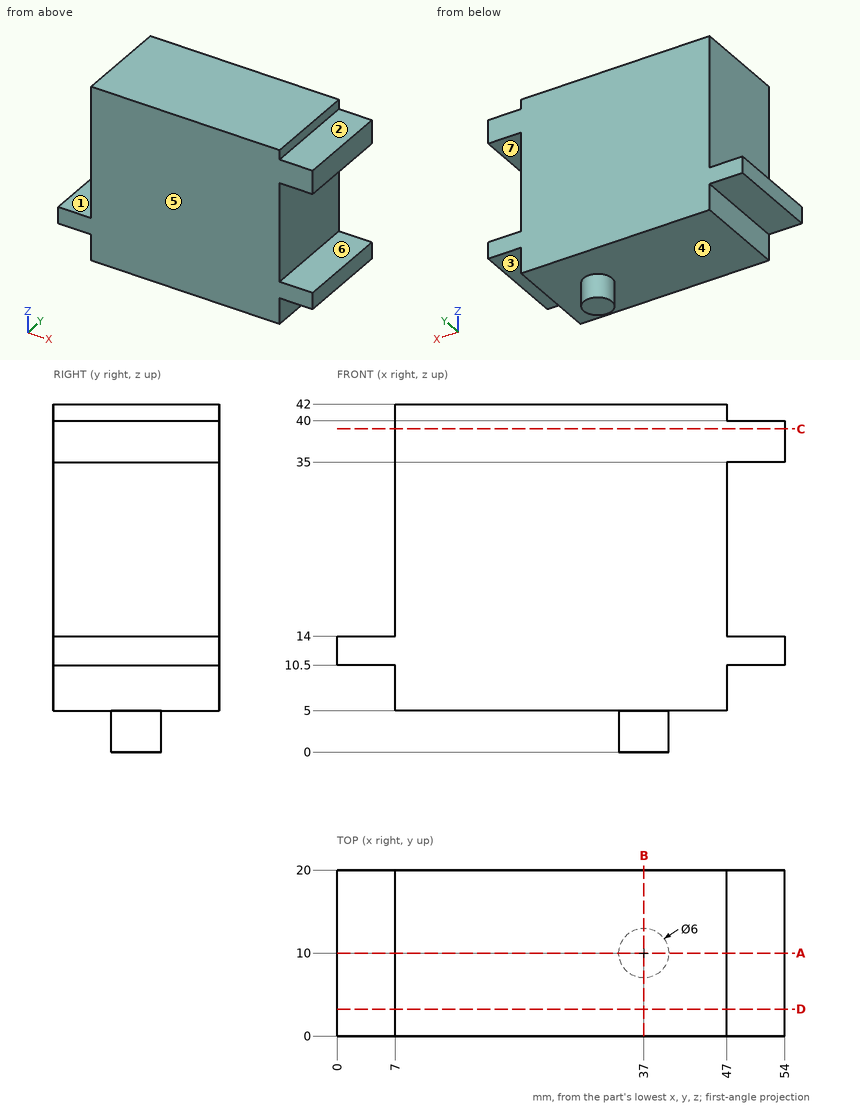
Answer from the drawing. Dimensions are ordinates in mm from the lowest x, y and z of the part. A direction names the side the tool comes from. Coordinates: 2 decimals unless noted, no trailing zeros. Write each loop counter-clockwise with the first axis right and the second up, starting at its lowest first coordinate (ties: lowest second). Pieces come first, ordered by that corner, then holes. Notation, with made-up numbers: M -25.75,-34 L -18.75,-34 A32 cw -18.75,0 Z; hole C 82.5,-20.5 d1. An arc over 180 degrees is marked long. Use a Markdown table: item, result.
Q1. The part is cut by section A-A, the plane y = 10. Write down the section's boundary in (x, z).
Answer block:
| item | result |
|---|---|
| outline | M 0,10.5 L 7,10.5 L 7,5 L 34,5 L 34,0 L 40,0 L 40,5 L 47,5 L 47,10.5 L 54,10.5 L 54,14 L 47,14 L 47,35 L 54,35 L 54,40 L 47,40 L 47,42 L 7,42 L 7,14 L 0,14 Z |
Q2. Determine the mould class of the marked faces 4, 5, 6 and 7 for opening direction Z: released by +Z, released by -Z, zero draft, split by the parting line, or undercut.
Answer block:
| item | result |
|---|---|
| face 4 | released by -Z |
| face 5 | zero draft |
| face 6 | undercut |
| face 7 | undercut |
Q3. The part is cut by section D-D, the plane y = 3.25. Write down the section's boundary in (x, z), then the cut area to 3 significant figures.
Answer block:
| item | result |
|---|---|
| outline | M 0,10.5 L 7,10.5 L 7,5 L 47,5 L 47,10.5 L 54,10.5 L 54,14 L 47,14 L 47,35 L 54,35 L 54,40 L 47,40 L 47,42 L 7,42 L 7,14 L 0,14 Z |
| area | 1,560 mm2 |
Q4. Each of these flat-tipped pins is pushed along its axis until it touches: pin 1 Ø3.5 at (x, y) = (51.5, 11) entering from +Z; pin 2 Ø1 at (x, y) = (38.5, 3) entering from -Z; pin 3 Ø1.6 at (y, z) = (13.5, 8.5) entering from +X. Where does it stop, or does it pass through?
Answer block:
| item | result |
|---|---|
| pin 1 | stops at z = 40 |
| pin 2 | stops at z = 5 |
| pin 3 | stops at x = 47 |
Q5. Which of the six approach directions +Z, -Z, +X, -X, +Y, -Y give full straight-line access (tool end or side, diameter ignored) to the marked faces 1, 2 and 3?
Answer block:
| item | result |
|---|---|
| face 1 | +Z, -X, +Y, -Y |
| face 2 | +Z, +X, +Y, -Y |
| face 3 | -Z, +X, +Y, -Y |
Q6. Straight lines are drawn through the part: L1, parallel to Z at x = 48.5, y = 10.5; L2, parallel to X at y = 14.25, z = 33; L3, parallel to Z at x = 27.5, y = 13. For each, find the intervals that lie inside material, in ascending order. Write a range as [from, to].
Answer block:
| item | result |
|---|---|
| L1 | z = [10.5, 14], [35, 40] |
| L2 | x = [7, 47] |
| L3 | z = [5, 42] |
Q7. The part is cut by section B-B, the plane x = 37. Write down the section's boundary in (y, z), then the cut area to 3 significant figures.
Answer block:
| item | result |
|---|---|
| outline | M 0,5 L 7,5 L 7,0 L 13,0 L 13,5 L 20,5 L 20,42 L 0,42 Z |
| area | 770 mm2 |
Q8. The part is cut by section C-C, the plane z = 39. Write down the section's boundary in (x, y), then the cut area to 3 significant figures.
Answer block:
| item | result |
|---|---|
| outline | M 7,0 L 54,0 L 54,20 L 7,20 Z |
| area | 940 mm2 |
